The model under review builds one solid part; all positions refer to its coordinate system, in mm. A direction names the side the tool comes from. Round coordinates to 2 decimals unless told otherwise and drop trailing zeros. Loops run counter-clockwise (first coordinate to the right, second up) from the corner with the lowest first, then second, coordinate; pieces in that order, holes last. Notation, with made-up numbers: (42.5, -16) -> (49.5, -16) arc R20 ccw to (49.5, -9) -> close; hole circle Ø3 at (8, 63). An arc over 180 degrees is marked (long way). Use a Markdown table: item, result. Add a question column.
1) Mouldability with a two-part tool opening along Z and no side actions: class faces 1 (the flat face through (66, -3, 4.762)), 2 (the cylindrical face through (54.599, -3.131, -5.256)), 3 (the flat face through (32, 0, 0)) as released by +Z, released by -Z, zero draft, split by the parting line, or undercut.
2) Consider section B-B on x = 15. Give the boundary of the cut face in (y, z), plus the area to 3 significant figures.
3) For faces 4 (the flat face through (26, -3, 4.775)), 5 (the flat face through (32, -6.35, 0)), 6 (the flat face through (66, -3, -4.762)), 7 (the flat face through (26, -3, -4.775)), list the 3-axis set-ups (+Z, -Z, +X, -X, +Y, -Y) from which the entire face can be reached by the end or side of a thin tool; tool diameter is ignored.
4) Wall thickness on probe 1 along Z at (x, y) = (46.5, -2); probe 2 along Z at (x, y) = (65.5, -4.5); probe 3 along Z at (x, y) = (62, -3.5): over which ranges is each line inside the solid? List them lowest first.
5) Insertion check: pin 1 (1.7 mm diameter, centred on x = 66.5, y = -4.5, fed in from -Z); pin 2 (1.5 mm diameter, centred on y = -1, z = -6.5, fed in from -X); pin 3 (3 mm diameter, centred on x = 36.5, y = -4, fed in from +Z); pin 4 (1.5 mm diameter, centred on x = 32.5, z = -7, fed in from +Y). Each pin has a flat end and moves straight along its axis. Give the tip position at first contact, or say it passes through.
6) Consider section C-C on z = 3. Give the boundary of the cut face in (x, y).
from build123d import *

# Parameters (mm, degrees)
F1_DEPTH = 6.35


with BuildPart() as f1:
    # F0 (on Front) → F1 (new body)
    with BuildSketch(Plane.XZ):
        with BuildLine():
            Line((52.175445, 4.7752), (0, 4.7752))
            ThreePointArc((0, 4.7752), (-4.7752, 0), (0, -4.7752))
            Line((0, -4.7752), (52.175445, -4.7752))
            ThreePointArc((52.175445, -4.7752), (54.631508, -5.269412), (56.705267, -6.67512))
            ThreePointArc((56.705267, -6.67512), (63.295562, -9.522806), (70.001999, -6.960577))
            ThreePointArc((70.001999, -6.960577), (70.316497, -5.566537), (69.135066, -4.7625))
            Line((69.135066, -4.7625), (63.5, -4.7625))
            ThreePointArc((63.5, -4.7625), (60.132404, -3.367596), (58.7375, 0))
            ThreePointArc((58.7375, 0), (60.132404, 3.367596), (63.5, 4.7625))
            Line((63.5, 4.7625), (69.135066, 4.7625))
            ThreePointArc((69.135066, 4.7625), (70.316497, 5.566537), (70.001999, 6.960577))
            ThreePointArc((70.001999, 6.960577), (63.295562, 9.522806), (56.705267, 6.67512))
            ThreePointArc((56.705267, 6.67512), (54.631508, 5.269412), (52.175445, 4.7752))
        make_face()
    extrude(amount=F1_DEPTH)


solid = f1.part
Result set:
| question | item | result |
|---|---|---|
| 1 | face 1 | undercut |
| 1 | face 2 | released by -Z |
| 1 | face 3 | zero draft |
| 2 | outline | (-6.35, -4.78) -> (0, -4.78) -> (0, 4.78) -> (-6.35, 4.78) -> close |
| 2 | area | 60.6 mm2 |
| 3 | face 4 | +Z, -X, +Y, -Y |
| 3 | face 5 | +Z, -Z, +X, -X, -Y |
| 3 | face 6 | +X, +Y, -Y |
| 3 | face 7 | -Z, -X, +Y, -Y |
| 4 | probe 1 | -4.78 to 4.78 |
| 4 | probe 2 | -9.31 to -4.76, 4.76 to 9.31 |
| 4 | probe 3 | -9.41 to -4.52, 4.52 to 9.41 |
| 5 | pin 1 | z = -9.28 |
| 5 | pin 2 | x = 55.56 |
| 5 | pin 3 | z = 4.78 |
| 5 | pin 4 | through |
| 6 | outline | (-3.72, -6.35) -> (59.8, -6.35) -> (59.8, 0) -> (-3.72, 0) -> close |
